Can you work these out from the model? Positions are in its coordinate system, mm. Face numbers are marked on the shaded views. A direction names the side the tool comes from. Give positions to 0.01 mm unless a question says otherwise; leave off trailing zeros. Order: outer loops, then holes, each group sorted by start corner. A loop starts at its lowest first (then second) coordinate and runs counter-clockwise, first axis right, second up. Notation, with made-up numbers: (-34.5, -40) - (8.5, -40) arc R32 cw to (8.5, -9) - close; hole circle Ø4 at (66, -26.75). An arc over 180 degrees is marked (long way). Answer as a JSON object with one key per item and string values.
```python
from build123d import *

# Parameters (mm, degrees)
CUT_EXTRUDE1_REACH          = 63.3
SKETCH8_R                   = 1.75
TAP_DRILL_FOR_M3_TAP2_D     = 2.5
TAP_DRILL_FOR_M3_TAP2_DEPTH = 6
TAP_DRILL_FOR_M3_TAP2_TIP   = 0.751075774
TAP_DRILL_FOR_M6_TAP1_D     = 5
TAP_DRILL_FOR_M6_TAP1_DEPTH = 10
TAP_DRILL_FOR_M6_TAP1_TIP   = 1.502151548
CUT_EXTRUDE2_REACH          = 63.3
FILLET1_R                   = 1
CUT_EXTRUDE3_REACH          = 41.749
SKETCH18_R                  = 1


with BuildPart() as part:
    # Sketch3 → Revolve1 (revolve)
    with BuildSketch(Plane.XY):
        Polygon((208.551545348, -139.573704322), (250.685153788, -139.573704322), (259.301545348, -139.573704322), (259.301545348, -133.573704322), (238.427343436, -133.573704322), (221.801545348, -133.573704322), (221.801545348, -131.073704322), (198.001545348, -131.073704322), (198.001545348, -133.573704322), (198.001545348, -140.556086521), (198.001545348, -145.198704322), (205.151545348, -145.198704322), (205.151545348, -140.573704322), (208.551545348, -140.573704322), align=None)
    revolve(axis=Axis((227.370475166, -148.573704322, 0), (1, 0, 0)))

    # Sketch8 → Cut-Extrude1 (cut, up to next)
    with BuildSketch(Plane(origin=(259.301545348, 0, 0), x_dir=(0, 0, -1), z_dir=(1, 0, 0)), mode=Mode.PRIVATE) as cut_extrude1_sk1:
        with Locations((0, -136.573704322)):
            Circle(SKETCH8_R)
    cut_extrude1_tool1 = extrude(cut_extrude1_sk1.sketch, amount=-CUT_EXTRUDE1_REACH, mode=Mode.PRIVATE) & part.part
    add(cut_extrude1_tool1.solids().sort_by_distance((259.301545, -136.573704, 0))[0], mode=Mode.SUBTRACT)
    # Sketch8 → Cut-Extrude1 (cut, up to next)
    with BuildSketch(Plane(origin=(259.301545348, 0, 0), x_dir=(0, 0, -1), z_dir=(1, 0, 0)), mode=Mode.PRIVATE) as cut_extrude1_sk2:
        with Locations((0, -160.573704322)):
            Circle(SKETCH8_R)
    cut_extrude1_tool2 = extrude(cut_extrude1_sk2.sketch, amount=-CUT_EXTRUDE1_REACH, mode=Mode.PRIVATE) & part.part
    add(cut_extrude1_tool2.solids().sort_by_distance((259.301545, -160.573704, 0))[0], mode=Mode.SUBTRACT)

    # Tap Drill for M3 Tap2
    with Locations(Plane(origin=(259.301545348, 0, 0), x_dir=(0, 0, -1), z_dir=(1, 0, 0))):
        with Locations((-12, -148.573704322), (12, -148.573704322)):
            Hole(TAP_DRILL_FOR_M3_TAP2_D / 2, depth=TAP_DRILL_FOR_M3_TAP2_DEPTH)
            with Locations((0, 0, -(TAP_DRILL_FOR_M3_TAP2_DEPTH + TAP_DRILL_FOR_M3_TAP2_TIP / 2))):  # 118° drill point
                Cone(0, TAP_DRILL_FOR_M3_TAP2_D / 2, TAP_DRILL_FOR_M3_TAP2_TIP, mode=Mode.SUBTRACT)

    # Tap Drill for M6 Tap1
    with Locations(Plane.ZY.offset(-198.001545348)):
        with Locations((12, -148.573704322), (-12, -148.573704322)):
            Hole(TAP_DRILL_FOR_M6_TAP1_D / 2, depth=TAP_DRILL_FOR_M6_TAP1_DEPTH)
            with Locations((0, 0, -(TAP_DRILL_FOR_M6_TAP1_DEPTH + TAP_DRILL_FOR_M6_TAP1_TIP / 2))):  # 118° drill point
                Cone(0, TAP_DRILL_FOR_M6_TAP1_D / 2, TAP_DRILL_FOR_M6_TAP1_TIP, mode=Mode.SUBTRACT)

    # Sketch16 → Cut-Extrude2 (cut, up to next)
    with BuildSketch(Plane.ZY.offset(-198.001545348), mode=Mode.PRIVATE) as cut_extrude2_sk1:
        Polygon((-16.98037611, -144.340876996), (-4.232827326, -131.593328212), (-6.354147669, -129.472007869), (-19.101696453, -142.219556653), align=None)
    cut_extrude2_tool1 = extrude(cut_extrude2_sk1.sketch, amount=-CUT_EXTRUDE2_REACH, mode=Mode.PRIVATE) & part.part
    add(cut_extrude2_tool1.solids().sort_by_distance((198.001545, -136.906442, -11.667262))[0], mode=Mode.SUBTRACT)
    # Sketch16 → Cut-Extrude2 (cut, up to next)
    with BuildSketch(Plane.ZY.offset(-198.001545348), mode=Mode.PRIVATE) as cut_extrude2_sk2:
        Polygon((4.232827326, -165.554080432), (6.354147669, -167.675400776), (19.101696453, -154.927851992), (16.98037611, -152.806531648), align=None)
    cut_extrude2_tool2 = extrude(cut_extrude2_sk2.sketch, amount=-CUT_EXTRUDE2_REACH, mode=Mode.PRIVATE) & part.part
    add(cut_extrude2_tool2.solids().sort_by_distance((198.001545, -160.240966, 11.667262))[0], mode=Mode.SUBTRACT)

    # Fillet1
    fillet1_edges = [part.edges().sort_by_distance(p)[0] for p in [
        (209.901545348, -152.806531648, 16.98037611),
        (209.901545348, -165.554080432, 4.232827326),
        (209.901545348, -144.340876996, -16.98037611),
        (209.901545348, -131.593328212, -4.232827326),
    ]]
    fillet(fillet1_edges, radius=FILLET1_R)

    # Sketch18 → Cut-Extrude3 (cut, up to next)
    with BuildSketch(Plane(origin=(0, -289.84438159, -120.057473832), x_dir=(1, 0, 0), z_dir=(0, 0.707106781, -0.707106781)), mode=Mode.PRIVATE) as cut_extrude3_sk1:
        with Locations((231.801545348, -184.786907758)):
            Circle(SKETCH18_R)
    cut_extrude3_tool1 = extrude(cut_extrude3_sk1.sketch, amount=CUT_EXTRUDE3_REACH, mode=Mode.PRIVATE) & part.part
    add(cut_extrude3_tool1.solids().sort_by_distance((231.801545, -159.180306, 10.606602))[0], mode=Mode.SUBTRACT)


solid = part.part
```
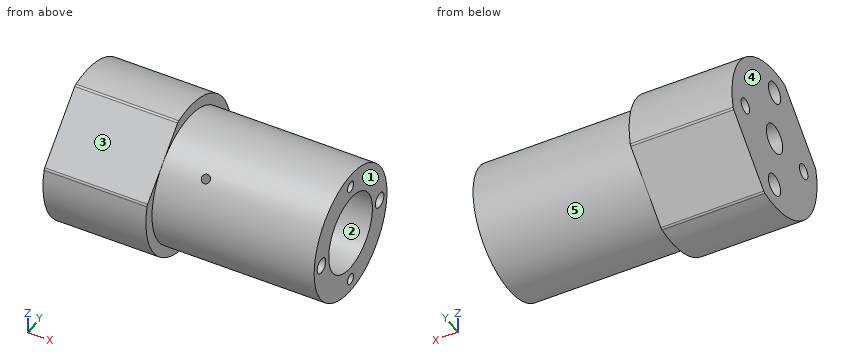
Q1. We'd pull the mould along Z, two halves only. Please class the marked faces 1, 2 and 3: released by +Z, released by -Z, zero draft, split by the parting line, or undercut.
Recorded:
{"face 1": "zero draft", "face 2": "undercut", "face 3": "released by +Z"}
Q2. If we section it at A-A, the plane z = 0: Please give me the cut outline in (x, y), then the cut area to 3 significant figures.
Recorded:
{"outline": "(198, -166.07) - (221.8, -166.07) - (221.8, -163.57) - (259.3, -163.57) - (259.3, -162.32) - (198, -162.32) - close; (198, -158.82) - (259.3, -158.82) - (259.3, -157.57) - (208.55, -157.57) - (208.55, -156.57) - (205.15, -156.57) - (205.15, -151.95) - (198, -151.95) - close; (198, -145.2) - (205.15, -145.2) - (205.15, -140.57) - (208.55, -140.57) - (208.55, -139.57) - (259.3, -139.57) - (259.3, -138.32) - (198, -138.32) - close; (198, -134.82) - (259.3, -134.82) - (259.3, -133.57) - (221.8, -133.57) - (221.8, -131.07) - (198, -131.07) - close", "area": "513 mm^2"}
Q3. I'm going to push flat-ended pins straight in: pin 1 Ø3 at (x, z) = (251.5, 5) entering from +Y; pin 2 Ø3 at (y, z) = (-148.57, 12) entering from -X; pin 3 Ø11 at (y, z) = (-148.57, 0) entering from +X. Where does each tip first touch, or does it pass through?
Recorded:
{"pin 1": "stops at y = -133.99", "pin 2": "stops at x = 208.6", "pin 3": "stops at x = 205.15"}
Q4. Which directions (+Z, -Z, +X, -X, +Y, -Y) give clear straight access to the entire face, cutting with the end or side of a thin tool? Please do the marked faces 4 and 5.
Recorded:
{"face 4": "+Z, -Z, -X, +Y, -Y", "face 5": "+X"}
Q5. If we section it at C-C, the plane y = -143.5: Please give me the cut outline in (x, z), then the cut area to 3 significant figures.
Recorded:
{"outline": "(198, -16.14) - (221.8, -16.14) - (221.8, -14.12) - (259.3, -14.12) - (259.3, -7.43) - (208.55, -7.43) - (208.55, -6.19) - (205.15, -6.19) - (205.15, 6.19) - (208.55, 6.19) - (208.55, 7.43) - (259.3, 7.43) - (259.3, 14.12) - (221.8, 14.12) - (221.8, 16.75) - (198, 16.75) - close", "area": "1,040 mm^2"}
Q6. I need wall thicknesses on L1, parallel to Y at x = 235, z = -1; L2, parallel to Y at x = 223, z = 3; L3, parallel to X at y = -156.5, z = 13. Which ranges of each line are inside material? Lowest first, please.
Recorded:
{"L1": "y = -163.54 to -162.01, -159.14 to -157.52, -139.63 to -138.01, -135.14 to -133.61", "L2": "y = -163.27 to -157.06, -140.09 to -133.88", "L3": "x = 198 to 221.8"}
Q7. If we section it at B-B, the plane x = 210.5: Please give me the cut outline in (y, z).
Recorded:
{"outline": "(-165.62, 3.95) arc R17.5 ccw to (-144.62, -17.05) arc R1 ccw to (-144.14, -16.78) - (-131.79, -4.43) arc R1 ccw to (-131.53, -3.95) arc R17.5 ccw to (-152.52, 17.05) arc R1 ccw to (-153.01, 16.78) - (-165.35, 4.43) arc R1 ccw to start; hole circle Ø3.5 at (-160.57, 0); hole circle Ø18 at (-148.57, 0); hole circle Ø3.5 at (-136.57, 0)"}
Q8. If we section it at D-D, the plane x = 240: Please give me the cut outline in (y, z), then the cut area to 3 significant figures.
Recorded:
{"outline": "circle Ø30 at (-148.57, 0); hole circle Ø3.5 at (-160.57, 0); hole circle Ø18 at (-148.57, 0); hole circle Ø3.5 at (-136.57, 0)", "area": "433 mm^2"}
